Could you check a few things on this model? Use its own coordinates, in mm. A direction names the side the tool comes from. Give positions to 0.01 mm unless a question says otherwise; leave off trailing zeros. Write each loop counter-clockwise with the first axis right and the second up, starting at its lowest first coordinate (ties: lowest second). Pieces come first, ordered by that corner, then holes. Notation, with made-up numbers: M 84.5,-2 L 134.5,-2 A35 cw 134.5,36 Z; hole C 74.25,18.5 d11. An arc over 180 degrees is marked long. One line per item, written item: value.
```python
from build123d import *

# Parameters (mm, degrees)
BOSS_EXTRUDE1_DEPTH = 9
BOSS_EXTRUDE2_DEPTH = 6.1
SKETCH3_W           = 11.33
SKETCH3_H           = 5
CUT_EXTRUDE1_DEPTH  = 10
SKETCH4_W           = 15
SKETCH4_H           = 3.533
CUT_EXTRUDE2_DEPTH  = 0.9
SKETCH5_W           = 15
SKETCH5_H           = 3.533
CUT_EXTRUDE3_DEPTH  = 2


with BuildPart() as part:
    # Sketch1 → Boss-Extrude1 (new body)
    with BuildSketch(Plane(origin=(0, 0, 0), x_dir=(1, 0, 0), z_dir=(0, 1, 0))):
        with BuildLine():
            Line((0, 4.6665), (5, 4.6665))
            ThreePointArc((5, 4.6665), (9.6665, 0), (5, -4.6665))
            Line((5, -4.6665), (0, -4.6665))
            ThreePointArc((0, -4.6665), (-4.6665, 0), (0, 4.6665))
        make_face()
        with BuildLine():
            Line((0, 3.2665), (5, 3.2665))
            ThreePointArc((5, 3.2665), (8.2665, 0), (5, -3.2665))
            Line((5, -3.2665), (0, -3.2665))
            ThreePointArc((0, -3.2665), (-3.2665, 0), (0, 3.2665))
        make_face(mode=Mode.SUBTRACT)
    extrude(amount=BOSS_EXTRUDE1_DEPTH)

    # Sketch2 → Boss-Extrude2 (add)
    with BuildSketch(Plane(origin=(0, 2, 0), x_dir=(1, 0, 0), z_dir=(0, 1, 0))):
        with BuildLine():
            Line((0, 3.2665), (5, 3.2665))
            ThreePointArc((5, 3.2665), (8.2665, 0), (5, -3.2665))
            Line((5, -3.2665), (0, -3.2665))
            ThreePointArc((0, -3.2665), (-3.2665, 0), (0, 3.2665))
        make_face()
        with BuildLine():
            Line((0, 2.8665), (5, 2.8665))
            ThreePointArc((5, 2.8665), (7.8665, 0), (5, -2.8665))
            Line((5, -2.8665), (0, -2.8665))
            ThreePointArc((0, -2.8665), (-2.8665, 0), (0, 2.8665))
        make_face(mode=Mode.SUBTRACT)
    extrude(amount=BOSS_EXTRUDE2_DEPTH)

    # Sketch3 → Cut-Extrude1 (cut)
    with BuildSketch(Plane.XY.offset(4.6665)):
        with Locations((2.5, 5)):
            Rectangle(SKETCH3_W, SKETCH3_H)
    extrude(amount=-CUT_EXTRUDE1_DEPTH, mode=Mode.SUBTRACT)

    # Sketch4 → Cut-Extrude2 (cut)
    with BuildSketch(Plane(origin=(0, 9, 0), x_dir=(1, 0, 0), z_dir=(0, 1, 0))):
        with Locations((2.5, 0.5)):
            Rectangle(SKETCH4_W, SKETCH4_H)
    extrude(amount=-CUT_EXTRUDE2_DEPTH, mode=Mode.SUBTRACT)

    # Sketch5 → Cut-Extrude3 (cut)
    with BuildSketch(Plane.XZ):
        with Locations((2.5, -0.5)):
            Rectangle(SKETCH5_W, SKETCH5_H)
    extrude(amount=-CUT_EXTRUDE3_DEPTH, mode=Mode.SUBTRACT)


solid = part.part
```
1) We'd pull the mould along Y, two halves only. Please class faces 1 (the face through (3, 0, -4)), 2 (the face through (-3.165, 5, 0)), 3 (the face through (2.5, 8.5, 3.266)): pulls with the +Y half, pulls with the -Y half, needs draft (parallel to the pull), parting line crosses it, or undercut.
Outcome:
face 1: pulls with the -Y half
face 2: undercut
face 3: needs draft
2) Please list where these lines run through material, in increasing order: L1, parallel to X at y = 3.25, z = -1.25 (3 decimals); L2, parallel to Z at x = 3, y = 1.5; L3, parallel to Y at x = 7, z = -4. Write a range as from..to.
Outcome:
L1: x = -4.496..-3.165, 8.165..9.496
L2: z = -4.67..-3.27, 3.27..4.67
L3: y = 0..2.5, 7.5..9
3) If we section it at C-C, the plane x = 3.5: Write out the boundary of the cut face in (y, z).
Outcome:
outline: M 0,-4.67 L 2.5,-4.67 L 2.5,-2.87 L 2,-2.87 L 2,-3.27 L 0,-3.27 Z; M 0,3.27 L 2,3.27 L 2,2.87 L 2.5,2.87 L 2.5,4.67 L 0,4.67 Z; M 7.5,-4.67 L 9,-4.67 L 9,-3.27 L 8.1,-3.27 L 8.1,-2.87 L 7.5,-2.87 Z; M 7.5,2.87 L 8.1,2.87 L 8.1,3.27 L 9,3.27 L 9,4.67 L 7.5,4.67 Z
4) If we section it at A-A, the plane y = 8.5: Write out the boundary of the cut face in (x, z), then the cut area to 3 significant figures.
Outcome:
outline: M -4.49,1.27 L -3.01,1.27 A3.27 cw 0,3.27 L 5,3.27 A3.27 cw 8.01,1.27 L 9.49,1.27 A4.67 ccw 5,4.67 L 0,4.67 A4.67 ccw Z; M -4.08,-2.27 A4.67 ccw 0,-4.67 L 5,-4.67 A4.67 ccw 9.08,-2.27 L 7.35,-2.27 A3.27 cw 5,-3.27 L 0,-3.27 A3.27 cw -2.35,-2.27 Z
area: 38.5 mm^2
5) I'm going to push flat-ended pins straight in: pin 1 (2 mm diameter, centred on x = 6, z = -0.5, fed in from +Y); pin 2 (0.5 mm diameter, centred on x = 8, y = 0.5, fed in from +Z); pin 3 (3 mm diameter, centred on x = 7.5, y = 5, fed in from +Z). Where does each tip first touch, or does it pass through?
Outcome:
pin 1: passes through
pin 2: stops at z = 3.77
pin 3: stops at z = 3.43
6) On a 3-axis mill with a long thin cutter (end or side, diameter ignored), from which of +Z, -Z, +X, -X, +Y, -Y can I reach the whole of each face in a straight line? I mean faces 4 (the face through (7.866, 7.796, -0.063)), 5 (the face through (-1.78, 8.54, 2.74)), 6 (the face through (2.4, 2.5, 3.2)). Say none if no direction works.
Outcome:
face 4: +Y, -Y
face 5: +Y
face 6: +Z, -Z
7) If we section it at D-D, the plane z = 1.5: Write out the boundary of the cut face in (x, y) (3 decimals), then the cut area to 3 significant figures.
Outcome:
outline: M -4.419,0 L -2.902,0 L -2.902,2 L -2.443,2 L -2.443,2.5 L -3.165,2.5 L -3.165,7.5 L -2.443,7.5 L -2.443,8.1 L -2.902,8.1 L -2.902,9 L -4.419,9 Z; M 7.443,2 L 7.902,2 L 7.902,0 L 9.419,0 L 9.419,9 L 7.902,9 L 7.902,8.1 L 7.443,8.1 L 7.443,7.5 L 8.165,7.5 L 8.165,2.5 L 7.443,2.5 Z
area: 25.7 mm^2
